The figure shows three views and two pictorial views of one solid part (mm, origin at its lowest corner). Answer the questions. A direction names the side the tool comes from. Coordinates: 2 decimals unless noted, no trailing zeros. Write each loop counter-clockwise with the first axis right and the second up, starting at its lowest first coordinate (ties: lowest second). Pieces come first, ordered by that corner, then holes.
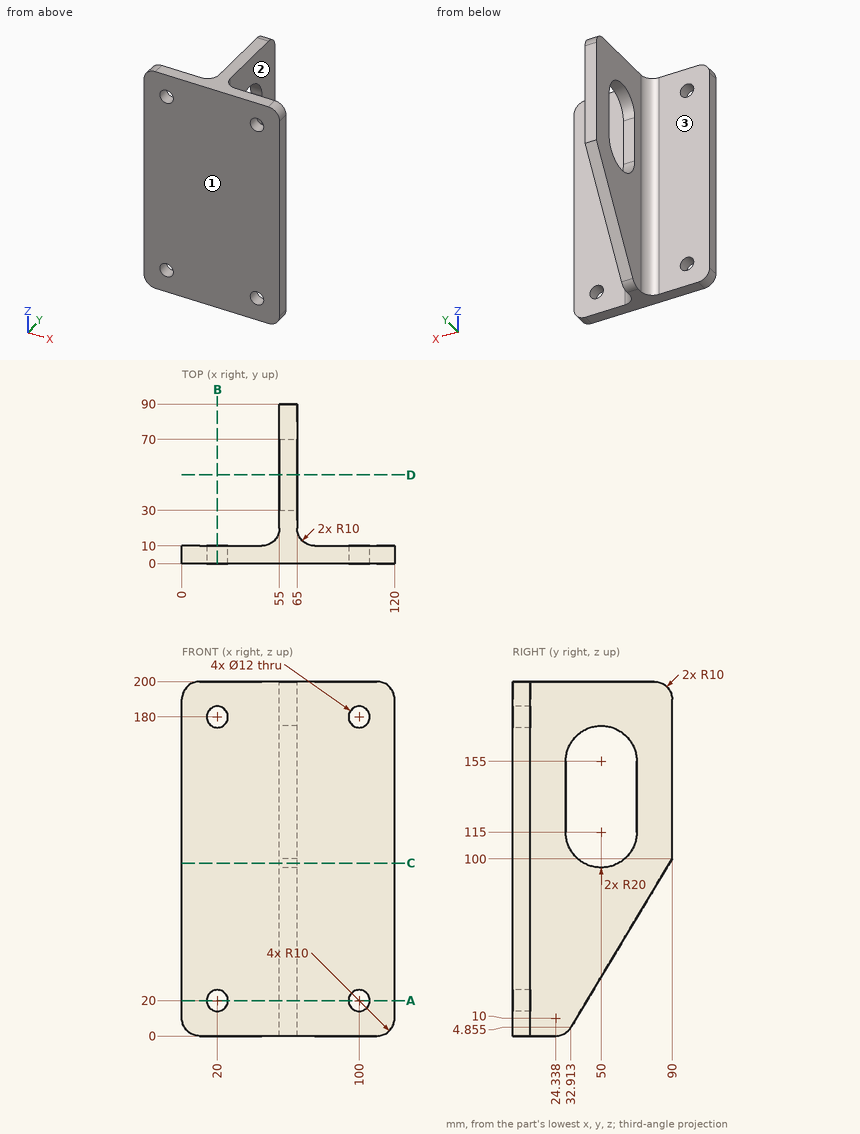
Q1. The part is cut by section C-C, the plane z = 97.5. Write down the section's boundary in (x, y), then the cut area to 3 significant figures.
Answers below:
outline: (0, 0) - (120, 0) - (120, 10) - (75, 10) arc R10 cw to (65, 20) - (65, 40.32) - (55, 40.32) - (55, 20) arc R10 cw to (45, 10) - (0, 10) - close; (55, 59.68) - (65, 59.68) - (65, 88.5) - (55, 88.5) - close
area: 1,830 mm2
Q2. Find the intervals of material crossed by probe 1 along Z at (x, y) = (100, 5.75); probe 2 along Y at (x, z) = (61.5, 122.5); probe 3 along Y at (x, z) = (85.5, 18), in increasing order.
Answers below:
probe 1: z = 0 to 14, 26 to 174, 186 to 200
probe 2: y = 0 to 30, 70 to 90
probe 3: y = 0 to 10
Q3. Which of the six approach directions +Z, -Z, +X, -X, +Y, -Y give full straight-line access (tool end or side, diameter ignored) to the marked faces 1, 2 and 3?
Answers below:
face 1: +Z, -Z, +X, -X, -Y
face 2: +Z, -Z, +X, +Y
face 3: +Z, -Z, -X, +Y
Q4. The part is cut by section B-B, the plane x = 20. Write down the section's boundary in (y, z).
Answers below:
outline: (0, 0) - (10, 0) - (10, 14) - (0, 14) - close; (0, 26) - (10, 26) - (10, 174) - (0, 174) - close; (0, 186) - (10, 186) - (10, 200) - (0, 200) - close
Q5. Given pin 1 (8 mm diameter, centred on y = 45.5, z = 30, fed in from -X); pin 2 (1.5 mm diameter, centred on x = 103.5, z = 120.5, fed in from +Y); pin 3 (4 mm diameter, centred on x = 45.5, z = 122.5, fed in from +Y), each flat-ended and moving along its own axis, determine where each tip first touches the part or whether it passes through.
Answers below:
pin 1: stops at x = 55
pin 2: stops at y = 10
pin 3: stops at y = 10.32
Q6. The part is cut by section D-D, the plane y = 50. Write down the section's boundary in (x, z).
Answers below:
outline: (55, 33.33) - (65, 33.33) - (65, 95) - (55, 95) - close; (55, 175) - (65, 175) - (65, 200) - (55, 200) - close
Q7. The part is cut by section A-A, the plane z = 20. Write down the section's boundary in (x, y), then the cut area to 3 significant figures.
Answers below:
outline: (0, 0) - (14, 0) - (14, 10) - (0, 10) - close; (26, 0) - (94, 0) - (94, 10) - (75, 10) arc R10 cw to (65, 20) - (65, 42) - (55, 42) - (55, 20) arc R10 cw to (45, 10) - (26, 10) - close; (106, 0) - (120, 0) - (120, 10) - (106, 10) - close
area: 1,320 mm2
